from build123d import *

# Parameters (mm, degrees)
F3_DEPTH = 22
F4_COUNT = 6


with BuildPart() as f1:
    # F0 (on Front) → F1 (revolve)
    with BuildSketch(Plane.XZ):
        with BuildLine():
            Line((-3.5, 12), (-56, 12))
            ThreePointArc((-56, 12), (-58.8284271247, 10.8284271247), (-60, 8))
            Line((-60, 8), (-60, -9.1715728753))
            ThreePointArc((-60, -9.1715728753), (-59.69551813, -10.7023066047), (-58.8284271247, -12))
            Line((-58.8284271247, -12), (-56, -12))
            Line((-56, -12), (-57.4142135624, -10.5857864376))
            ThreePointArc((-57.4142135624, -10.5857864376), (-57.847759065, -9.93693974), (-58, -9.1715728753))
            Line((-58, -9.1715728753), (-58, 8))
            ThreePointArc((-58, 8), (-57.4142135624, 9.4142135624), (-56, 10))
            Line((-56, 10), (-5.5, 10))
            Line((-5.5, 10), (-5.5, -12))
            Line((-5.5, -12), (-3.5, -12))
            Line((-3.5, -12), (-3.5, 12))
        make_face()
    revolve(axis=Axis((0, 0, 0), (0, 0, 1)))

    # F2 (on face) → F3 (join, through all)
    with BuildSketch(Plane(origin=(0, 0, 10), x_dir=(1, 0, 0), z_dir=(0, 0, -1))):
        with BuildLine():
            ThreePointArc((1, -55.9910707167), (0, -56), (-1, -55.9910707167))
            Line((-1, -55.9910707167), (-1, -57.9913786696))
            ThreePointArc((-1, -57.9913786696), (0, -58), (1, -57.9913786696))
            Line((1, -57.9913786696), (1, -55.9910707167))
        make_face()
        with BuildLine():
            ThreePointArc((1, -5.4083269132), (0, -5.5), (-1, -5.4083269132))
            Line((-1, -5.4083269132), (-1, -55.9910707167))
            ThreePointArc((-1, -55.9910707167), (0, -56), (1, -55.9910707167))
            Line((1, -55.9910707167), (1, -5.4083269132))
        make_face()
    extrude(amount=F3_DEPTH)

    # F4: F1 ×6 about axis
    f4_axis = Axis((0, 0, 0), (0, 0, 1))


with BuildPart() as f1_1:
    add(f1.part)
    for i in range(1, F4_COUNT):
        add(f1.part.rotate(f4_axis, i * 360 / F4_COUNT))


solid = f1_1.part
Geometry check sheet. Reference: the model listing, model coordinates, mm. A direction names the side the tool comes from. Round coordinates to 2 decimals unless told otherwise and drop trailing zeros. Order: outer loops, then holes, each group sorted by start corner. A loop starts at its lowest first (then second) coordinate and runs counter-clockwise, first axis right, second up. Notation, with made-up numbers: (27, -18.5) - (69, -18.5) arc R29 ccw to (69, 8.5) - close; hole circle Ø1 at (-2, -5.75). An arc over 180 degrees is marked (long way). One line per question, with ' | ' between items. Start each with the question number.
(1) Access from +Z, -Z, +X, -X, +Y, -Y to the whole of each face (thin tool, end or side, straight path). Record for faces 1 (the conical face through (-28.47, -48.51, -11.75)), 2 (the flat face through (-36, 0, 10)), 3 (the cylindrical face through (-3.233, 1.341, 0.168)).
(2) Thickness scan on L1, parallel to Y at x = 0, z = 6.75; L2, parallel to X at y = 51.5, z = 3.75; L3, parallel to X at y = -18, z = -9.5. Record the ranges inside material, lowest first. Write a range as [from, to].
(3) Sectioned sample at A-A on z = 4.25. Record the cut outline in (x, y), and give its area (3 significant figures).
(4) Depth check by flat-ended pin: pin 1 Ø6.5 at (y, z) = (-44, -2.5) entering from -X; pin 2 Ø2 at (y, z) = (-42, 6) entering from -X; pin 3 Ø6.5 at (y, z) = (-30.5, 1.5) entering from +X (3 decimals). Enter the tip coordinate at first touch or a pass-through.
(5) Release check for a two-part mould opening along Z. For faces 4 (the cylindrical face through (-58, 0, 0)), 5 (the flat face through (20, 29, 10)), 6 (the cylindrical face through (5.5, 0, -1.2)) record: released by +Z, released by -Z, zero draft, split by the parting line, or undercut.
Conclusion:
1) face 1: none | face 2: -Z | face 3: +Z, -Z
2) L1: y = [-60, -3.5], [3.5, 60] | L2: x = [-30.79, -26.68], [-1, 1], [26.68, 30.79] | L3: x = [-57.22, -55.11], [-33.18, -29.18], [-1, 1], [29.18, 33.18], [55.11, 57.22]
3) outline: circle Ø120 at (0, 0); hole (-50.72, -28.13) - (-5.18, -1.84) arc R5.5 cw to (-5.18, 1.84) - (-50.72, 28.13) arc R58 ccw to start; hole (-49.72, -29.86) arc R58 ccw to (-1, -57.99) - (-1, -5.41) arc R5.5 cw to (-4.18, -3.57) - close; hole (-49.72, 29.86) - (-4.18, 3.57) arc R5.5 cw to (-1, 5.41) - (-1, 57.99) arc R58 ccw to start; hole circle Ø7 at (0, 0); hole (1, -57.99) arc R58 ccw to (49.72, -29.86) - (4.18, -3.57) arc R5.5 cw to (1, -5.41) - close; hole (1, 5.41) arc R5.5 cw to (4.18, 3.57) - (49.72, 29.86) arc R58 ccw to (1, 57.99) - close; hole (5.18, -1.84) - (50.72, -28.13) arc R58 ccw to (50.72, 28.13) - (5.18, 1.84) arc R5.5 cw to start | area: 1,430 mm2
4) pin 1: stops at x = -44.04 | pin 2: stops at x = -43.81 | pin 3: stops at x = 53.455
5) face 4: undercut | face 5: released by -Z | face 6: zero draft
